Geometry check sheet. Reference: drawing and pictorial views, mm from the part's lowest x, y, z. A direction names the side the tool comes from. Give positions to 0.01 mm unless a question says otherwise; leave off trailing zeros. Loops run counter-clockwise (first coordinate to the right, second up) from the corner with the lowest first, then second, coordinate; pieces in that order, holes last. Notation, with made-up numbers: (-24, 50) -> (24, 50) arc R27 ccw to (24, 68) -> close; hole circle Ø2 at (51, -25.75). An arc over 180 degrees is marked (long way). One line per item, written item: value. Start each with the question number.
(1) Sectioned sample at B-B, the plane y = 3. Record the cut outline in (x, z), then the cut area to 3 significant figures.
(2) Sectioned sample at A-A, the plane z = 20.5. Record the cut outline in (x, y).
(3) Tool access check on the marked faces 1, 2, 3 and 4. Record the directions out of +Z, -Z, +X, -X, +Y, -Y that give a thin tool (end or side, any length) a straight path to the whole face; none if there is none.
(4) Gauge pin test, flat ends, axial feed: pin 1 Ø1.2 at (x, y) = (49.5, 20) entering from +Z; pin 2 Ø1 at (y, z) = (4, 35) entering from +X (3 decimals); pin 3 Ø3 at (y, z) = (3.5, 19) entering from +X. Record the tip position at first contact, or that the pin passes through.
(5) Sectioned sample at D-D, the plane x = 24. Record the cut outline in (y, z).
(6) Scan lines: line 1 along X through (y, z) = (5.5, 27); line 2 along X through (y, z) = (17.25, 2); line 3 along Z through (x, y) = (27.5, 5.5). Record each from-to range of solid material in increasing order. Write a range as from..to.
(7) Sectioned sample at C-C, the plane x = 33. Record the cut outline in (y, z), then the cut area to 3 significant figures.
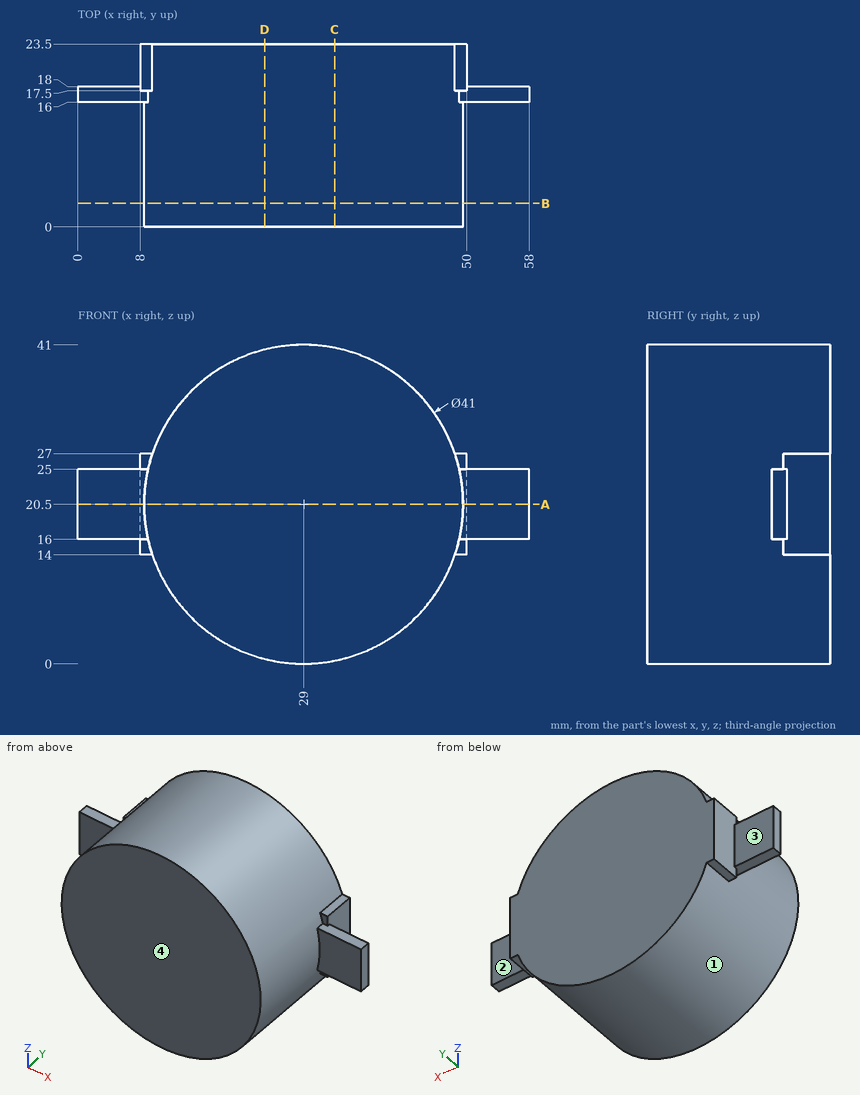
Calculated:
1. outline: circle Ø41 at (29, 20.5)
1. area: 1,320 mm2
2. outline: (0, 16) -> (8.5, 16) -> (8.5, 0) -> (49.5, 0) -> (49.5, 16) -> (58, 16) -> (58, 18) -> (50, 18) -> (50, 23.5) -> (8, 23.5) -> (8, 18) -> (0, 18) -> close
3. face 1: -Y
3. face 2: +Z, -Z, +X, +Y
3. face 3: +Z, -Z, -X, +Y
3. face 4: +Z, -Z, +X, -X, -Y
4. pin 1: stops at z = 27
4. pin 2: stops at x = 43.975
4. pin 3: stops at x = 49.5
5. outline: (0, 0.62) -> (23.5, 0.62) -> (23.5, 40.38) -> (0, 40.38) -> close
6. line 1: x = 9.56..48.44
6. line 2: x = 20.17..37.83
6. line 3: z = 0.05..40.95
7. outline: (0, 0.39) -> (23.5, 0.39) -> (23.5, 40.61) -> (0, 40.61) -> close
7. area: 945 mm2
